Build history of the part. All positions in model axes, mm. A direction names the side the tool comes from. Round coordinates to 2 decimals unless told otherwise and drop trailing zeros. Write each loop counter-clockwise with the first axis right and the second up, starting at its lowest first coordinate (ties: lowest second). Pieces come first, ordered by that corner, then holes.
Item 1: Wall check: probe 1 along Y at (x, z) = (-138.25, -2.05); probe 2 along X at (y, z) = (-1.5, -1.6); probe 3 along Y at (x, z) = (-145.5, -1.65). Give the ranges that are in metal, low to high.
Item 2: Drop flat-ended pins along their axis: pin 1 Ø1.5 at (y, z) = (12, -1) entering from -X; pin 2 Ø7.5 at (x, y) = (-136.5, 10) entering from +Z. Give the stop position or say it passes through.
Item 3: Mould opens along X. For faces 3 (the flat face through (-147.6, -3.2, -1.5)), 4 (the flat face through (-127.6, 8.1, -1.5)), 5 (the cylindrical face through (-129.824, 22.166, -1.479)), 6 (the cylindrical face through (-129.45, 26.9, -1.48)) say: +X half, -X half, draft (parallel to the pull), parting line (faces both ways), or undercut.
Item 4: Band-saw the part on A-A, the plane z = -0.65. Write the cut outline in (x, y), then the cut area to 3 significant figures.
Item 5: Band-saw the part on B-B, the plane x = -127.75. Write the cut outline in (y, z), then the cut area to 3 significant figures.
Item 6: 3-axis set-ups, long thin cutter, end or side, ignore diameter. For faces 1 (the cylindrical face through (-155.43, 8.43, -1.48)), 2 (the cylindrical face through (-136.321, 3.655, -1.232)): which of +Z, -Z, +X, -X, +Y, -Y reach the whole face in a straight line?
Autodesk Inventor part; units mm, degrees
ref_plane "YZ Plane" through (0, 0, 0) normal (1, 0, 0) x (0, 1, 0)
ref_plane "XZ Plane" through (0, 0, 0) normal (0, 1, 0) x (-1, 0, 0)
ref_plane "XY Plane" through (0, 0, 0) normal (0, 0, 1) x (1, 0, 0)
sketch "スケッチ1" plane through (0, 0, 0) normal (0, 0, 1) x (1, 0, 0)
  circle A0 centre (-132.6852, 21.2646) radius 3
  circle A1 centre (-105.2485, 37.922) radius 3
  circle A2 centre (-84.1159, 33.5789) radius 3
  circle A3 centre (-77.8119, 54.5794) radius 3
  circle A4 centre (-112.1063, 12.5661) radius 3
  circle A5 centre (-136.4636, -3.8437) radius 3
  circle A6 centre (-147.9517, 7.8722) radius 3
  line L0 (-62.3105, 66.9855) -> (-56.4162, 71.4105)
  line L1 (-56.4162, 71.4105) -> (-60.2332, 71.5281)
  arc A7 (-60.2332, 71.5281) -> (-64.0951, 70.5113) centre (-60.4494, 64.5064) ccw
  line L2 (-64.0951, 70.5113) -> (-153.1544, 16.4415)
  arc A8 (-153.1544, 16.4415) -> (-154.1888, 0.0236) centre (-147.9517, 7.8722) ccw
  line L3 (-154.1888, 0.0236) -> (-141.4408, -10.1069)
  arc A9 (-141.4408, -10.1069) -> (-131.6607, -10.2415) centre (-136.4636, -3.8437) ccw
  line L4 (-131.6607, -10.2415) -> (-40.2316, 58.3956)
  arc A10 (-40.2316, 58.3956) -> (-37.5466, 65.3193) centre (-44.4492, 64.0137) ccw
  line L5 (-37.5466, 65.3193) -> (-62.5812, 46.5254)
  arc A11 (-66.3034, 51.4837) -> (-62.5812, 46.5254) centre (-64.4423, 49.0046) ccw
  line L6 (-66.3034, 51.4837) -> (-41.2688, 70.2776)
  arc A12 (-41.2688, 70.2776) -> (-44.233, 71.0354) centre (-44.4492, 64.0137) ccw
  line L7 (-44.233, 71.0354) -> (-46.496, 71.105)
  line L8 (-46.496, 71.105) -> (-58.5883, 62.0272)
  arc A13 (-62.3105, 66.9855) -> (-58.5883, 62.0272) centre (-60.4494, 64.5064) ccw
  circle A14 centre (-147.9517, 7.8722) radius 1.5
  circle A15 centre (-147.9517, 7.8722) radius 7.5
  circle A16 centre (-136.4636, -3.8437) radius 1.5
  circle A17 centre (-136.4636, -3.8437) radius 7.5
  circle A18 centre (-132.6852, 21.2646) radius 1.5
  circle A19 centre (-132.6852, 21.2646) radius 6.5
  line L9 (-152.6141, 13.7469) -> (-136.7259, 26.3561)
  line L10 (-126.2244, 20.5513) -> (-129.0089, -4.6668)
  line L11 (-153.3068, 2.6212) -> (-141.8187, -9.0947)
  point P0 (0, 0)
  point P1 (0, 0)
  dimension "d0" = 15
  dimension "d1" = 15
extrude "押し出し1" add sketch "スケッチ1" against normal blind 3 contours A19 | A19 L10 A17 L11 A15 L9 | A15 | A17
sketch "スケッチ2" plane through (0, 0, 0) normal (0, 0, 1) x (1, 0, 0)
  arc A0 (-152.6141, 13.7469) -> (-153.3068, 2.6212) centre (-147.9517, 7.8722) ccw
  line L0 (-153.3068, 2.6212) -> (-141.8187, -9.0947)
  arc A1 (-141.8187, -9.0947) -> (-129.0089, -4.6668) centre (-136.4636, -3.8437) ccw
  line L1 (-129.0089, -4.6668) -> (-126.2244, 20.5513)
  arc A2 (-126.2244, 20.5513) -> (-136.7259, 26.3561) centre (-132.6852, 21.2646) ccw
  line L2 (-136.7259, 26.3561) -> (-152.6141, 13.7469)
  circle A3 centre (-136.4636, -3.8437) radius 3
  circle A4 centre (-132.6852, 21.2646) radius 3
  circle A5 centre (-147.9517, 7.8722) radius 3
  line L3 (-129.2063, 20.8805) -> (-131.9908, -4.3375)
  arc A6 (-139.6766, -6.9943) -> (-131.9908, -4.3375) centre (-136.4636, -3.8437) ccw
  line L4 (-139.6766, -6.9943) -> (-151.1648, 4.7216)
  arc A7 (-150.7491, 11.397) -> (-151.1648, 4.7216) centre (-147.9517, 7.8722) ccw
  line L5 (-150.7491, 11.397) -> (-134.8609, 24.0062)
  arc A8 (-129.2063, 20.8805) -> (-134.8609, 24.0062) centre (-132.6852, 21.2646) ccw
  arc A9 (-152.6141, 13.7469) -> (-153.3068, 2.6212) centre (-147.9517, 7.8722) ccw
  circle A10 centre (-147.9517, 7.8722) radius 7.5
  circle A11 centre (-132.6852, 21.2646) radius 6.5
  circle A12 centre (-136.4636, -3.8437) radius 7.5
  point P0 (0, 0)
  point P1 (-143.8774, -2.7102)
  point P2 (-131.3323, 1.6262)
  point P3 (-129.8074, 15.4364)
  point P4 (-139.1512, 20.6013)
  point P5 (-146.0493, 15.1269)
  point P6 (-146.964, 0.4375)
  dimension "d4" = 3
extrude "押し出し2" cut sketch "スケッチ2" against normal blind 2.5 contours L5 A11 L3 A12 L4 A10
sketch "スケッチ3" plane through (0, 0, 0) normal (0, 0, 1) x (1, 0, 0)
  arc A0 (-146.964, 0.4375) -> (-146.0493, 15.1269) centre (-147.9517, 7.8722) ccw
  line L0 (-146.0493, 15.1269) -> (-139.1512, 20.6013)
  arc A1 (-139.1512, 20.6013) -> (-129.8074, 15.4364) centre (-132.6852, 21.2646) ccw
  line L1 (-129.8074, 15.4364) -> (-131.3323, 1.6262)
  arc A2 (-131.3323, 1.6262) -> (-143.8774, -2.7102) centre (-136.4636, -3.8437) ccw
  line L2 (-143.8774, -2.7102) -> (-146.964, 0.4375)
  arc A3 (-152.6141, 13.7469) -> (-153.3068, 2.6212) centre (-147.9517, 7.8722) ccw
  line L3 (-153.3068, 2.6212) -> (-141.8187, -9.0947)
  arc A4 (-141.8187, -9.0947) -> (-129.0089, -4.6668) centre (-136.4636, -3.8437) ccw
  line L4 (-129.0089, -4.6668) -> (-126.2244, 20.5513)
  arc A5 (-126.2244, 20.5513) -> (-136.7259, 26.3561) centre (-132.6852, 21.2646) ccw
  line L5 (-136.7259, 26.3561) -> (-152.6141, 13.7469)
  circle A6 centre (-136.4636, -3.8437) radius 3
  circle A7 centre (-132.6852, 21.2646) radius 3
  circle A8 centre (-147.9517, 7.8722) radius 3
  arc A9 (-142.9322, -0.048) -> (-144.2837, 1.3303) centre (-143.7947, 0.4581) ccw
  arc A10 (-141.4831, 4.0765) -> (-140.1316, 2.6982) centre (-140.6207, 3.5704) ccw
  point P0 (0, 0)
  dimension "d7" = 2
  dimension "d8" = 2
extrude "押し出し3" add sketch "スケッチ3" against normal blind 3 contours A0 A10 A2 A9
fillet "フィレット1" radius 1 6 edges at (-146.964, 0.4375, -1.25) (-143.8774, -2.7102, -1.25) (-146.0493, 15.1269, -1.25) (-139.1512, 20.6013, -1.25) (-129.8074, 15.4364, -1.25) (-131.3323, 1.6262, -1.25)
properties part number "アーム 中間節 先端中詰め" material "ポリカーボネート、クリア"
Results:
1. probe 1: y = -11.13 to -6.25, -1.43 to 3.44, 17.91 to 25.15
1. probe 2: x = -149.27 to -145.06, -143.71 to -138.34, -134.59 to -128.66
1. probe 3: y = -5.34 to -1.06, 0.77 to 6.14, 9.6 to 19.39
2. pin 1: stops at x = -154.65
2. pin 2: stops at z = -2.5
3. face 3: -X half
3. face 4: +X half
3. face 5: undercut
3. face 6: parting line
4. outline: (-153.31, 2.62) - (-141.82, -9.09) arc R7.5 ccw to (-129.01, -4.67) - (-126.22, 20.55) arc R6.5 ccw to (-136.73, 26.36) - (-152.61, 13.75) arc R7.5 ccw to start; hole circle Ø6 at (-147.95, 7.87); hole (-145.74, -0.81) - (-145.1, -1.46) arc R1 ccw to (-143.45, -1.13) arc R7.5 cw to (-142.93, -0.05) arc R1 ccw to (-144.28, 1.33) arc R7.5 cw to (-145.37, 0.83) arc R1 ccw to start; hole (-144.68, 16.21) arc R1 ccw to (-144.52, 14.54) arc R7.5 cw to (-141.48, 4.08) arc R1 ccw to (-140.13, 2.7) arc R7.5 cw to (-132.64, 2.61) arc R1 ccw to (-131.14, 3.36) - (-129.98, 13.85) arc R1 ccw to (-131.2, 14.94) arc R6.5 cw to (-138.83, 19.15) arc R1 ccw to (-140.4, 19.61) - close; hole circle Ø6 at (-136.46, -3.84); hole circle Ø6 at (-132.69, 21.26)
4. area: 522 mm2
5. outline: (6.73, -3) - (25.49, -3) - (25.49, 0) - (6.73, 0) - close
5. area: 56.3 mm2
6. face 1: +Z, -Z, -X
6. face 2: +Z
